```python
from build123d import *

# Parameters (mm, degrees)
SKETCH1_W           = 101.6
SKETCH1_H           = 38.1
BOSS_EXTRUDE1_DEPTH = 19.05
SKETCH2_R           = 3.175
CUT_EXTRUDE1_DEPTH  = 16.51
CUT_EXTRUDE2_REACH  = 40.1
SKETCH3_R           = 3.429
SKETCH4_R           = 13.335
CUT_EXTRUDE3_DEPTH  = 16.51
SKETCH5_R           = 3.556
CUT_EXTRUDE4_DEPTH  = 20.05
SKETCH6_W           = 20.32
SKETCH6_H           = 5.08
CUT_EXTRUDE5_DEPTH  = 15.24


with BuildPart() as part:
    # Sketch1 → Boss-Extrude1 (new body)
    with BuildSketch(Plane(origin=(0, 0, 0), x_dir=(1, 0, 0), z_dir=(0, 1, 0))):
        with Locations((12.918491372, -8.273443983)):
            Rectangle(SKETCH1_W, SKETCH1_H)
    extrude(amount=BOSS_EXTRUDE1_DEPTH)

    # Sketch2 → Cut-Extrude1 (cut)
    with BuildSketch(Plane(origin=(0, 19.05, 0), x_dir=(1, 0, 0), z_dir=(0, 1, 0))):
        with Locations((-27.721508628, 0.616556017)):
            Circle(SKETCH2_R)
        with Locations((53.558491372, 0.616556017)):
            Circle(SKETCH2_R)
    extrude(amount=-CUT_EXTRUDE1_DEPTH, mode=Mode.SUBTRACT)

    # Sketch3 → Cut-Extrude2 (cut, up to next)
    with BuildSketch(Plane.XY.offset(27.323443983), mode=Mode.PRIVATE) as cut_extrude2_sk1:
        with Locations((-5.877508628, 9.525)):
            Circle(SKETCH3_R)
    cut_extrude2_tool1 = extrude(cut_extrude2_sk1.sketch, amount=-CUT_EXTRUDE2_REACH, mode=Mode.PRIVATE) & part.part
    add(cut_extrude2_tool1.solids().sort_by_distance((-5.877509, 9.525, 27.323444))[0], mode=Mode.SUBTRACT)
    # Sketch3 → Cut-Extrude2 (cut, up to next)
    with BuildSketch(Plane.XY.offset(27.323443983), mode=Mode.PRIVATE) as cut_extrude2_sk2:
        with Locations((31.714491372, 9.525)):
            Circle(SKETCH3_R)
    cut_extrude2_tool2 = extrude(cut_extrude2_sk2.sketch, amount=-CUT_EXTRUDE2_REACH, mode=Mode.PRIVATE) & part.part
    add(cut_extrude2_tool2.solids().sort_by_distance((31.714491, 9.525, 27.323444))[0], mode=Mode.SUBTRACT)

    # Sketch4 → Cut-Extrude3 (cut)
    with BuildSketch(Plane(origin=(0, 19.05, 0), x_dir=(1, 0, 0), z_dir=(0, 1, 0))):
        with Locations((12.918491372, -8.273443983)):
            Circle(SKETCH4_R)
    extrude(amount=-CUT_EXTRUDE3_DEPTH, mode=Mode.SUBTRACT)

    # Sketch5 → Cut-Extrude4 (cut, through all)
    with BuildSketch(Plane(origin=(0, 19.05, 0), x_dir=(1, 0, 0), z_dir=(0, 1, 0))):
        with Locations((12.918491372, -8.273443983)):
            Circle(SKETCH5_R)
    extrude(amount=-CUT_EXTRUDE4_DEPTH, mode=Mode.SUBTRACT)

    # Sketch6 → Cut-Extrude5 (cut)
    with BuildSketch(Plane(origin=(0, 19.05, 0), x_dir=(1, 0, 0), z_dir=(0, 1, 0))):
        with Locations((-27.721508628, 8.236556017)):
            Rectangle(SKETCH6_W, SKETCH6_H)
        with Locations((53.558491372, 8.236556017)):
            Rectangle(SKETCH6_W, SKETCH6_H)
    extrude(amount=-CUT_EXTRUDE5_DEPTH, mode=Mode.SUBTRACT)


solid = part.part
```
The model under review builds one solid part; all positions refer to its coordinate system, in mm. A direction names the side the tool comes from. Give positions to 0.01 mm unless a question says otherwise; leave off trailing zeros. Order: outer loops, then holes, each group sorted by start corner. A loop starts at its lowest first (then second) coordinate and runs counter-clockwise, first axis right, second up. Notation, with made-up numbers: (13, 67) - (64, 67) arc R17 ccw to (64, 81) - close; hole circle Ø4 at (60, 64). An arc over 180 degrees is marked (long way). Use CSV: the item, a comma, the result in double quotes. Start each with the question number.
Q1. To check wall thickness, follow line 1 along X through (y, z) = (7, 23); line 2 along X through (y, z) = (12, 1); line 3 along Z through (x, y) = (47, 12.5). State the ranges of each line that lie inside material, in increasing order. Write a range as [from, to].
Q2. Tool access review of faces 4 (the flat face through (53, 3.81, -8)), 5 (the cylindrical face through (-6.324, 12.925, 8.54)), 6 (the flat face through (-17.562, 12, -8)), 7 (the cylindrical face through (56.49, 10.91, 0.6)): name each direction out of +Z, -Z, +X, -X, +Y, -Y from which nothing blocks a thin tool from reaching the whole face with its end or side.
Q3. We need section A-A, the plane y = 10.5. State how many separate pieces and enclosed holes the cut face has, and give its area (3 significant figures).
Q4. The part is to be moulded in two halves that separate along Y. For faces 1 (the flat face through (63.718, 9, 9)), 2 (the flat face through (-28, 2.54, -1)), 3 (the cylindrical face through (29.187, 11.842, 8.54)), say which applies: +Y half, -Y half, draft (parallel to the pull), parting line (faces both ways), or undercut.
Q5. We need section B-B, the plane x = -7. Write out the cut boundary in (y, z), and give its area (3 significant figures).
Q6. Clearance check with flat-ended pins moving along their axes: pin 1 Ø21.5 at (x, z) = (12.92, 8.27) entering from +Y; pin 2 Ø1.5 at (y, z) = (8.5, -8) entering from +X; pin 3 Ø4.5 at (x, y) = (51, 13) entering from -Z. State where each tip first meets the part, or that it passes through.
Outcome:
1,line 1,"x = [-37.88, -8.2], [-3.56, 29.39], [34.03, 63.72]"
1,line 2,"x = [-37.88, -30.45], [-24.99, -8.25], [-3.5, 1.74], [24.1, 29.34], [34.09, 50.83], [56.29, 63.72]"
1,line 3,"z = [-5.7, 27.32]"
2,face 4,"-Z, +X, +Y"
2,face 5,"+Z, -Z"
2,face 6,"-Z, -X, +Y"
2,face 7,"+Y"
3,separate pieces,"3"
3,enclosed holes,"3"
3,area,"2,540 mm^2"
4,face 1,"draft"
4,face 2,"+Y half"
4,face 3,"undercut"
5,outline,"(0, -10.78) - (6.28, -10.78) - (6.28, 27.32) - (0, 27.32) - close; (12.77, -10.78) - (19.05, -10.78) - (19.05, 27.32) - (12.77, 27.32) - close"
5,area,"479 mm^2"
6,pin 1,"stops at y = 2.54"
6,pin 2,"stops at x = 43.4"
6,pin 3,"stops at z = -5.7"
